Autodesk Fusion 360 part; units mm, degrees
sketch "Sketch1" plane through (0, 0, 0) normal (1, 0, 0) x (0, 0, -1)
  line L0 (0, 12.45) -> (0, 14.875)
  line L1 (0, 14.875) -> (-16.51, 14.875)
  line L2 (-16.51, 14.875) -> (-16.51, 15.875)
  line L3 (-16.51, 15.875) -> (6.35, 15.875)
  line L4 (6.35, 15.875) -> (6.35, 17.78)
  line L5 (6.35, 17.78) -> (46.99, 17.78)
  line L6 (46.99, 17.78) -> (46.99, 12.5)
  line L7 (46.99, 12.5) -> (44.99, 12.5)
  line L8 (44.99, 12.5) -> (44.99, 0)
  line L9 (44.99, 0) -> (6.35, 0)
  line L10 (6.35, 0) -> (6.35, 14.875)
  line L11 (6.35, 14.875) -> (1, 14.875)
  line L12 (1, 14.875) -> (1, 12.45)
  line L13 (1, 12.45) -> (0, 12.45)
  dimension "d532" = 15.875
  dimension "d533" = 1
  dimension "d534" = 12.45
  dimension "d535" = 14.875
  dimension "d536" = 5.35
  dimension "d537" = 16.51
  dimension "d538" = 17.78
  dimension "d539" = 40.64
  dimension "d540" = 12.5
  dimension "d541" = 2
  dimension "d545" = 0
  dimension "d546" = 0
  dimension "d547" = 0
  dimension "d548" = 0
revolve "Revolve1" add sketch "Sketch1" angle 360 about axis through (0, 0, 1.75) along (0, 0, 1)
fillet "Fillet1" radius 1 2 edges at (-16.5768, 6.4295, -46.99) (-11.6541, 4.5202, -46.99)
equation "d532 = 1.25 in / 2"
properties part number "Eyepiece"
For this review, take the finished solid that the model builds, in its own axes (mm). A direction names the side the tool comes from. Round coordinates to 2 decimals unless told otherwise and drop trailing zeros. Loops run counter-clockwise (first coordinate to the right, second up) from the corner with the lowest first, then second, coordinate; pieces in that order, holes last. Notation, with made-up numbers: (52.5, -18) - (66.5, -18) arc R18 ccw to (66.5, 12) - close; hole circle Ø4 at (-6, -25.75). An arc over 180 degrees is marked (long way). Use one line per item in the form item = value.
1) We need section A-A on y = 0. Write out the cut boundary in (x, z) (3 decimals).
Solutions:
outline = (-17.78, -45.99) arc R1 ccw to (-16.78, -46.99) - (-13.5, -46.99) arc R1 ccw to (-12.5, -45.99) - (-12.5, -44.99) - (12.5, -44.99) - (12.5, -45.99) arc R1 ccw to (13.5, -46.99) - (16.78, -46.99) arc R1 ccw to (17.78, -45.99) - (17.78, -6.35) - (15.875, -6.35) - (15.875, 16.51) - (14.875, 16.51) - (14.875, 0) - (12.45, 0) - (12.45, -1) - (14.875, -1) - (14.875, -6.35) - (-14.875, -6.35) - (-14.875, -1) - (-12.45, -1) - (-12.45, 0) - (-14.875, 0) - (-14.875, 16.51) - (-15.875, 16.51) - (-15.875, -6.35) - (-17.78, -6.35) - close
2) We need section C-C on z = -42. Write out the cut boundary in (x, y).
Solutions:
outline = circle Ø35.56 at (0, 0)
3) Clearance check with flat-ended pins moving along their axes: P1, Ø3, axis at x = -4.5, z = -5, coming from the +Y side; P2, Ø6, axis at x = -3, z = -1, coming from the +Y side (3 decimals); P3, Ø15, axis at x = -3, y = -7, coming from the -Z side; P4, Ø10, axis at y = -7.5, z = -27.5, coming from the -X side. State where each tip first meets the part, or that it passes through.
Solutions:
P1 = 17.36
P2 = 15.875
P3 = -46.99
P4 = -17.6
4) Tool access review of faces 1 (the face through (0, 0, -44.99)), 2 (the face through (-8.41, -9.18, -0.49)), 3 (the face through (-12.54, 8, -3.64)): name each direction out of +Z, -Z, +X, -X, +Y, -Y from which nothing blocks a thin tool from reaching the whole face with its end or side.
Solutions:
face_1 = -Z
face_2 = +Z
face_3 = none
5) Wall thickness on probe 1 along X at (y, z) = (0, 5) (3 decimals); probe 2 along Z at (x, y) = (8, 12); probe 3 along X at (y, z) = (0, -0.4) (3 decimals): over which ranges is each line inside the solid? List them lowest first.
Solutions:
probe_1 = -15.875 to -14.875, 14.875 to 15.875
probe_2 = -46.99 to -6.35, -1 to 0
probe_3 = -15.875 to -12.45, 12.45 to 15.875
6) Mouldability with a two-part tool opening along Y and no side actions: class faces 4 (the face through (-17.36, -3.85, -26.45)), 5 (the face through (-3.755, 11.923, -45.483)), 6 (the face through (-12.54, 8, 8.37)), 7 (the face through (-15, -7, -6.35)) as pulls with the +Y half, pulls with the -Y half, needs draft (parallel to the pull), parting line crosses it, or undercut.
Solutions:
face_4 = parting line crosses it
face_5 = undercut
face_6 = undercut
face_7 = needs draft
7) We need section D-D on z = 4.5. Write out the cut boundary in (x, y) (3 decimals).
Solutions:
outline = circle Ø31.75 at (0, 0); hole circle Ø29.75 at (0, 0)
